Model file for the job. Use its own axes, mm. Face numbers are marked on the shaded views. A direction names the side the tool comes from. Round coordinates to 2 decimals unless told otherwise and drop trailing zeros. Loops run counter-clockwise (first coordinate to the right, second up) from the corner with the lowest first, then second, coordinate; pieces in that order, holes last. Notation, with made-up numbers: M -2.5,14.5 L 47.5,14.5 A16 cw 47.5,28.5 Z; hole C -9.75,30.25 d1. An arc over 180 degrees is marked long. Use a Markdown table: item, result. Add a question column.
Q1. Cut at A-A (z = -14.5). Give the cut face in (x, y).
Q2. Cut at D-D (y = 4.75). Give the cut face in (x, z).
Q3. Cut at C-C (z = 13.5). Give the cut face in (x, y), plus the area to 3 significant figures.
Q4. Pin check, flat tips, straight feed: pin 1 (5 mm diameter, centred on x = -13.13, y = 15, fed in from +Z); pin 2 (1.1 mm diameter, centred on x = -12.5, z = -16, fed in from -Y); pin 3 (1.6 mm diameter, centred on x = 17, y = 15.5, fed in from +Z); pin 4 (8 mm diameter, centred on x = 3.5, y = 14, fed in from +Z). Stop position of each tip, or through.
Q5. Cut at B-B (x = 17.5). Give the cut face in (y, z), plus the area to 3 significant figures.
Q6. Probe line 1 (X direction, y = 21.25, z = -4.5); line 2 (Z direction, x = -13, y = 17); line 3 (Z direction, x = 13.5, y = 6). List the from-to ranges inside material, lowest first. Write a range as from..to.
Q7. Mould opens along X. For the marked faces 3, 4 and 5 say: +X half, -X half, draft (parallel to the pull), parting line (faces both ways), or undercut.
Q8. Tool access for the marked faces 1 and 2: list every direction of +Z, -Z, +X, -X, +Y, -Y with a clear straight run to the whole face (end or side of a thin tool).
from build123d import *

# Parameters (mm, degrees)
BOSS_EXTRUDE1_DEPTH     = 30
CUT_EXTRUDE1_DEPTH      = 62.55558656
CUT_EXTRUDE1_DEPTH_BACK = 10
SKETCH4_R               = 1.5
CUT_EXTRUDE2_DEPTH      = 63.337896288
FILLET1_R               = 1.25
FILLET2_R               = 10
CUT_EXTRUDE3_DEPTH      = 1


with BuildPart() as part:
    # Sketch2 → Boss-Extrude1 (new body)
    with BuildSketch(Plane(origin=(0, 0, 0), x_dir=(1, 0, 0), z_dir=(0, 1, 0))):
        Polygon((26.115384615, 19.384615385), (-22.384615385, 19.384615385), (-22.384615385, -28.615384615), (-19.384615385, -28.615384615), (-19.384615385, 15.584615385), (23.115384615, 15.584615385), (23.115384615, -28.615384615), (26.115384615, -28.615384615), align=None)
    extrude(amount=BOSS_EXTRUDE1_DEPTH)

    # Sketch3 → Cut-Extrude1 (cut, two sides: drawn at the far end of the back side and taken through both)
    with BuildSketch(Plane(origin=(-19.384615385, 0, 0), x_dir=(0, 0, -1), z_dir=(1, 0, 0)).offset(-CUT_EXTRUDE1_DEPTH_BACK)):
        with BuildLine():
            ThreePointArc((-21.165384615, 10), (-17.723889294, 18.308504679), (-9.415384615, 21.75))
            Line((-9.415384615, 21.75), (-9.415384615, 24.25))
            ThreePointArc((-9.415384615, 24.25), (-19.491656247, 20.076271632), (-23.665384615, 10))
            Line((-23.665384615, 10), (-21.165384615, 10))
        make_face()
        with BuildLine():
            Line((-10.665384615, 10), (-9.415384615, 10))
            Line((-9.415384615, 10), (-9.415384615, 11.25))
            ThreePointArc((-9.415384615, 11.25), (-10.299268092, 10.883883476), (-10.665384615, 10))
        make_face()
        with BuildLine():
            Line((-9.415384615, 11.25), (-9.415384615, 10))
            Line((-9.415384615, 10), (-10.665384615, 10))
            ThreePointArc((-10.665384615, 10), (-9.415384615, 8.75), (-8.165384615, 10))
            ThreePointArc((-8.165384615, 10), (-8.531501139, 10.883883476), (-9.415384615, 11.25))
        make_face()
    extrude(amount=CUT_EXTRUDE1_DEPTH + CUT_EXTRUDE1_DEPTH_BACK, mode=Mode.SUBTRACT)

    # Sketch4 → Cut-Extrude2 (cut, through all)
    with BuildSketch(Plane(origin=(0, 0, -19.384615385), x_dir=(-1, 0, 0), z_dir=(0, 0, -1))):
        with Locations((-16.865384615, 15)):
            Circle(SKETCH4_R)
        with Locations((13.134615385, 15)):
            Circle(SKETCH4_R)
    extrude(amount=-CUT_EXTRUDE2_DEPTH, mode=Mode.SUBTRACT)

    # Fillet1
    fillet1_edges = [part.edges().sort_by_distance(p)[0] for p in [
        (-20.884615385, 24.25, 9.415384615),
        (-20.884615385, 21.75, 9.415384615),
        (-20.884615385, 10, 21.165384615),
        (-20.884615385, 10, 23.665384615),
        (24.615384615, 10, 23.665384615),
        (24.615384615, 10, 21.165384615),
        (24.615384615, 21.75, 9.415384615),
        (24.615384615, 24.25, 9.415384615),
    ]]
    fillet(fillet1_edges, radius=FILLET1_R - 0.0001)  # a hair under: the kernel refuses the full size

    # Fillet2
    fillet2_edges = [part.edges().sort_by_distance(p)[0] for p in [
        (-20.884615385, 30, 28.615384615),
        (24.615384615, 30, 28.615384615),
        (24.615384615, 0, 28.615384615),
        (-20.884615385, 0, 28.615384615),
    ]]
    fillet(fillet2_edges, radius=FILLET2_R)

    # Sketch5 → Cut-Extrude3 (cut)
    with BuildSketch(Plane.XY.offset(-15.584615385)):
        Polygon((-14.722328625, 12.25), (-11.546902144, 12.25), (-9.959188904, 15), (-11.546902144, 17.75), (-14.722328625, 17.75), (-16.310041865, 15), align=None)
        Polygon((15.277671375, 12.25), (18.453097856, 12.25), (20.040811096, 15), (18.453097856, 17.75), (15.277671375, 17.75), (13.689958135, 15), align=None)
    extrude(amount=-CUT_EXTRUDE3_DEPTH, mode=Mode.SUBTRACT)


solid = part.part
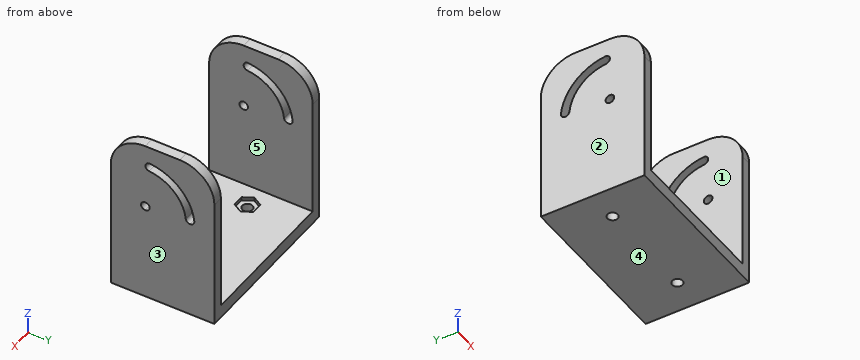
Checked values:
| question | item | result |
|---|---|---|
| 1 | outline | M -22.38,0 L -19.38,0 L -19.38,30 L -22.38,30 Z; M 23.12,0 L 26.12,0 L 26.12,30 L 23.12,30 Z |
| 2 | outline | M -22.38,-19.38 L 26.12,-19.38 L 26.12,27.13 L 23.12,27.13 L 23.12,-15.58 L -19.38,-15.58 L -19.38,27.13 L -22.38,27.13 Z |
| 3 | outline | M -22.38,0 L -19.38,0 L -19.38,21.02 L -22.38,21.02 Z; M -22.38,23.65 L -19.38,23.65 L -19.38,30 L -22.38,30 Z; M 23.12,0 L 26.12,0 L 26.12,21.02 L 23.12,21.02 Z; M 23.12,23.65 L 26.12,23.65 L 26.12,30 L 23.12,30 Z |
| 3 | area | 164 mm^2 |
| 4 | pin 1 | stops at z = -16.58 |
| 4 | pin 2 | stops at y = 0 |
| 4 | pin 3 | passes through |
| 4 | pin 4 | stops at z = -15.58 |
| 5 | outline | M 0,-19.38 L 13.64,-19.38 L 13.64,-16.58 L 12.25,-16.58 L 12.25,-15.58 L 0,-15.58 Z; M 16.36,-19.38 L 30,-19.38 L 30,-15.58 L 17.75,-15.58 L 17.75,-16.58 L 16.36,-16.58 Z |
| 5 | area | 101 mm^2 |
| 6 | line 1 | x = -22.38..-19.38, 23.12..26.12 |
| 6 | line 2 | z = -19.38..-16.58 |
| 6 | line 3 | z = -19.38..-15.58 |
| 7 | face 3 | +X half |
| 7 | face 4 | draft |
| 7 | face 5 | undercut |
| 8 | face 1 | +Z, +Y, -Y |
| 8 | face 2 | +Z, -Z, -X, +Y, -Y |
